Check sheet for the modelled part. Datum: model origin and axes. Units: mm. A direction names the side the tool comes from. Give positions to 0.01 mm unless a question says otherwise; leave off trailing zeros. Order: outer loops, then holes, each group sorted by start corner. A loop starts at its lowest first (then second) coordinate and runs counter-clockwise, first axis right, second up.
Item 1: Material ranges on line 1 along Y through (x, z) = (0, -2.5); line 2 along Y through (x, z) = (0, -0.2); line 3 along Y through (x, z) = (0, -8.25), recorded low to high.
Item 2: Sectioned sample at C-C on z = -11. Record the boundary of the cut face in (x, y), and give its area (3 significant figures).
Item 3: Access from +Z, -Z, +X, -X, +Y, -Y to the whole of each face (thin tool, end or side, straight path). Record for faces 5 (the cylindrical face through (16.453, 5.181, 0.394)), 6 (the flat face through (-7, -7, -2)).
Item 4: Release check for a two-part mould opening along X. For faces 1 (the cylindrical face through (0.27, 4.78, -2.04)), 2 (the flat face through (4, 0, 1)), 3 (the cylindrical face through (0.54, -2.44, -6.5)), 4 (the cylindrical face through (0.867, -3.905, -9.437)) record: released by +X, released by -X, zero draft, split by the parting line, or undercut.
Item 5: Sectioned sample at A-A on y = 0. Record the boundary of the cut face in (x, z), and give its area (3 significant figures).
Item 6: Sectioned sample at B-B on x = 0. Count the separate pieces of the cut face and the enclosed holes in it, and give its area (3 significant figures).
Item 7: Gauge pin test, flat ends, axial feed: P1, Ø2, axis at x = 0, y = 6, coming from the -Z side; P2, Ø8, axis at x = -9.5, z = -2.5, coming from the +Y side. Record the tip position at first contact, or that the pin passes through.
from build123d import *

# Parameters (mm, degrees)
SKETCH1_R           = 17.25
BOSS_EXTRUDE1_DEPTH = 1
SKETCH2_R           = 17
BOSS_EXTRUDE2_DEPTH = 2
SKETCH3_R           = 9
BOSS_EXTRUDE3_DEPTH = 3
SKETCH4_R           = 4
BOSS_EXTRUDE4_DEPTH = 9
SKETCH5_R           = 2.5
CUT_EXTRUDE1_DEPTH  = 29.637824638
SKETCH6_R           = 1.25
CUT_EXTRUDE2_DEPTH  = 27.002403735
CHAMFER1_SIZE       = 0.2


with BuildPart() as part:
    # Sketch1 → Boss-Extrude1 (new body)
    with BuildSketch(Plane.XY):
        Circle(SKETCH1_R)
    extrude(amount=BOSS_EXTRUDE1_DEPTH)

    # Sketch2 → Boss-Extrude2 (add)
    with BuildSketch(Plane(origin=(0, 0, 0), x_dir=(-1, 0, 0), z_dir=(0, 0, -1))):
        Circle(SKETCH2_R)
    extrude(amount=BOSS_EXTRUDE2_DEPTH)

    # Sketch3 → Boss-Extrude3 (add)
    with BuildSketch(Plane(origin=(0, 0, -2), x_dir=(-1, 0, 0), z_dir=(0, 0, -1))):
        Circle(SKETCH3_R)
    extrude(amount=BOSS_EXTRUDE3_DEPTH)

    # Sketch4 → Boss-Extrude4 (add)
    with BuildSketch(Plane(origin=(0, 0, -5), x_dir=(-1, 0, 0), z_dir=(0, 0, -1))):
        Circle(SKETCH4_R)
    extrude(amount=BOSS_EXTRUDE4_DEPTH)

    # Sketch5 → Cut-Extrude1 (cut, through all)
    with BuildSketch(Plane(origin=(0, 0, -14), x_dir=(-1, 0, 0), z_dir=(0, 0, -1))):
        Circle(SKETCH5_R)
    extrude(amount=-CUT_EXTRUDE1_DEPTH, mode=Mode.SUBTRACT)

    # Sketch6 → Cut-Extrude2 (cut, through all)
    with BuildSketch(Plane(origin=(0, 0, -5), x_dir=(-1, 0, 0), z_dir=(0, 0, -1))):
        with Locations((0, 6)):
            Circle(SKETCH6_R)
    extrude(amount=-CUT_EXTRUDE2_DEPTH, mode=Mode.SUBTRACT)

    # Chamfer1
    chamfer1_edges = [part.edges().sort_by_distance(p)[0] for p in [
        (9, 0, -5),
        (2.5, 0, -14),
        (-17.25, 0, 1),
        (17, 0, -2),
    ]]
    chamfer(chamfer1_edges, length=CHAMFER1_SIZE)


solid = part.part
Report:
1. line 1: y = -9 to -2.5, 2.5 to 4.75, 7.25 to 9
1. line 2: y = -17 to -2.5, 2.5 to 4.75, 7.25 to 17
1. line 3: y = -4 to -2.5, 2.5 to 4
2. outline: circle Ø8 at (0, 0); hole circle Ø5 at (0, 0)
2. area: 30.6 mm2
3. face 5: +Z, -Z
3. face 6: -Z
4. face 1: undercut
4. face 2: zero draft
4. face 3: undercut
4. face 4: split by the parting line
5. outline: (-17.25, 0) - (-17, 0) - (-17, -1.8) - (-16.8, -2) - (-9, -2) - (-9, -4.8) - (-8.8, -5) - (-4, -5) - (-4, -14) - (-2.7, -14) - (-2.5, -13.8) - (-2.5, 1) - (-17.05, 1) - (-17.25, 0.8) - close; (2.5, -13.8) - (2.7, -14) - (4, -14) - (4, -5) - (8.8, -5) - (9, -4.8) - (9, -2) - (16.8, -2) - (17, -1.8) - (17, 0) - (17.25, 0) - (17.25, 0.8) - (17.05, 1) - (2.5, 1) - close
5. area: 153 mm2
6. separate pieces: 3
6. enclosed holes: 0
6. area: 138 mm2
7. P1: passes through
7. P2: stops at y = 16.06
